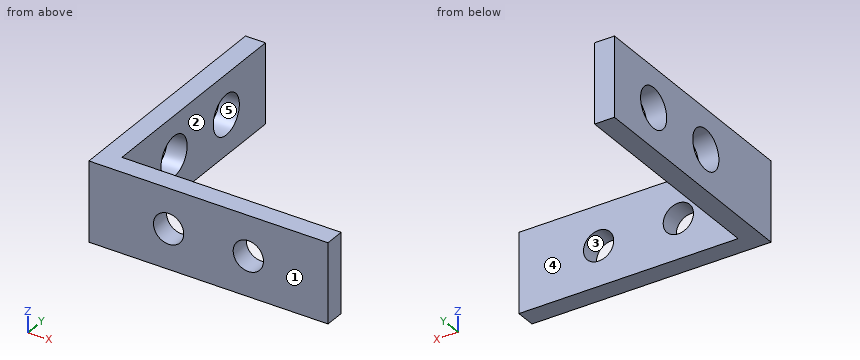
from build123d import *

# Parameters (mm, degrees)
BOSS_EXTRUDE1_DEPTH = 12.7
SKETCH2_R           = 2.413
CUT_EXTRUDE1_DEPTH  = 4.175
SKETCH3_R           = 3.175
CUT_EXTRUDE2_DEPTH  = 4.175


with BuildPart() as part:
    # Sketch1 → Boss-Extrude1 (new body)
    with BuildSketch(Plane.XY):
        Polygon((0, 0), (0, 38.1), (3.175, 38.1), (3.175, 3.175), (38.1, 3.175), (38.1, 0), align=None)
    extrude(amount=BOSS_EXTRUDE1_DEPTH)

    # Sketch2 → Cut-Extrude1 (cut, through all)
    with BuildSketch(Plane(origin=(0, 3.175, 0), x_dir=(1, 0, 0), z_dir=(0, 1, 0))):
        with Locations((12.7, -6.35)):
            Circle(SKETCH2_R)
        with Locations((25.4, -6.35)):
            Circle(SKETCH2_R)
    extrude(amount=-CUT_EXTRUDE1_DEPTH, mode=Mode.SUBTRACT)

    # Sketch3 → Cut-Extrude2 (cut, through all)
    with BuildSketch(Plane(origin=(3.175, 0, 0), x_dir=(0, 0, -1), z_dir=(1, 0, 0))):
        with Locations((-6.35, 28.575)):
            Circle(SKETCH3_R)
        with Locations((-6.35, 15.875)):
            Circle(SKETCH3_R)
    extrude(amount=-CUT_EXTRUDE2_DEPTH, mode=Mode.SUBTRACT)


solid = part.part
Input: part model. Units: mm. Frame: model coordinates. Face numbers are marked on the shaded views. A direction names the side the tool comes from. Give positions to 0.01 mm unless a question says otherwise; leave off trailing zeros. Write each loop counter-clockwise with the first axis right and the second up, starting at its lowest first coordinate (ties: lowest second). Pieces come first, ordered by that corner, then holes.
Q1. Section A-A, the plane x = 25.4. Output: boundary loops of the cut face in (y, z) (3 decimals).
Q2. Section B-B, the plane z = 6.35. Output: boundary loops of the cut face in (x, y) (3 decimals), plus the area to 3 significant figures.
Q3. Material intervals for probe 1 along X at (y, z) = (0.7, 6.35); probe 2 along Y at (x, z) = (2.2, 6.35); probe 3 along Z at (x, y) = (25.4, 2.3), sorted ascending.
Q4. Section D-D, the plane y = 7.5. Output: boundary loops of the cut face in (x, z) (3 decimals).
Q5. Set-up query: the marked faces 1 and 2. Return all of +Z, -Z, +X, -X, +Y, -Y with unobstructed straight access to the full face (end or side cutting, diameter ignored); none if empty.
Q6. First-contact query: P1, Ø4.5, axis at x = 12.7, z = 6.35, coming from the +Y side; P2, Ø3, axis at x = 9.5, z = 6, coming from the +Y side (3 decimals); P3, Ø3, axis at x = 32.5, z = 7.5, coming from the -Y side; P4, Ø6.5, axis at y = 18.5, z = 6, coming from the +X side (3 decimals). Flat tips, straight axial feed; report the tip coordinate or a pass-through.
Q7. Pull-direction query (Y, two-part tool) for the marked faces 3, 4 and 5; classes: pulls with the +Y half, pulls with the -Y half, needs draft (parallel to the pull), parting line crosses it, or undercut.
Q8. Section C-C, the plane y = 28. Output: boundary loops of the cut face in (x, z) (1 decimal), plus the area to 3 significant figures.
Filled in:
1. outline: (0, 0) - (3.175, 0) - (3.175, 3.937) - (0, 3.937) - close; (0, 8.763) - (3.175, 8.763) - (3.175, 12.7) - (0, 12.7) - close
2. outline: (0, 0) - (10.287, 0) - (10.287, 3.175) - (3.175, 3.175) - (3.175, 12.7) - (0, 12.7) - close; (0, 19.05) - (3.175, 19.05) - (3.175, 25.4) - (0, 25.4) - close; (0, 31.75) - (3.175, 31.75) - (3.175, 38.1) - (0, 38.1) - close; (15.113, 0) - (22.987, 0) - (22.987, 3.175) - (15.113, 3.175) - close; (27.813, 0) - (38.1, 0) - (38.1, 3.175) - (27.813, 3.175) - close
2. area: 161 mm2
3. probe 1: x = 0 to 10.29, 15.11 to 22.99, 27.81 to 38.1
3. probe 2: y = 0 to 12.7, 19.05 to 25.4, 31.75 to 38.1
3. probe 3: z = 0 to 3.94, 8.76 to 12.7
4. outline: (0, 0) - (3.175, 0) - (3.175, 12.7) - (0, 12.7) - close
5. face 1: +Z, -Z, +X, -X, -Y
5. face 2: +Z, -Z, +X, +Y
6. P1: passes through
6. P2: stops at y = 3.175
6. P3: stops at y = 0
6. P4: stops at x = 3.175
7. face 3: needs draft
7. face 4: pulls with the +Y half
7. face 5: undercut
8. outline: (0, 0) - (3.2, 0) - (3.2, 3.2) - (0, 3.2) - close; (0, 9.5) - (3.2, 9.5) - (3.2, 12.7) - (0, 12.7) - close
8. area: 20.5 mm2
